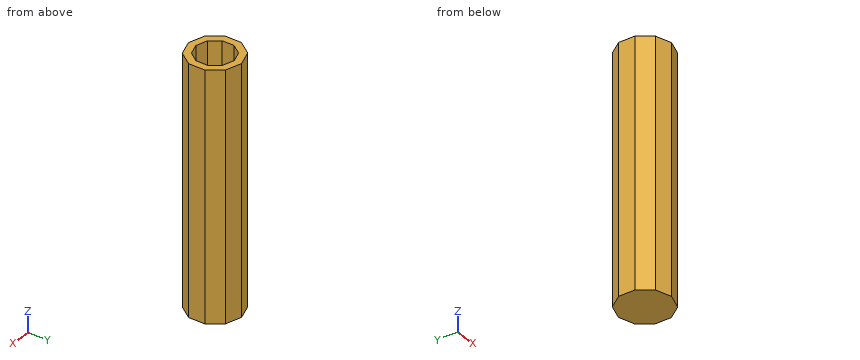
from build123d import *

# Parameters (mm, degrees)
F1_DEPTH = 381
F2_T     = -10.885714


with BuildPart() as f1:
    # F0 (on Top) → F1 (new body)
    with BuildSketch(Plane.XY):
        Polygon((39.086581, -12.7), (39.086581, 12.7), (24.156836, 33.249032), (0, 41.098063), (-24.156836, 33.249032), (-39.086581, 12.7), (-39.086581, -12.7), (-24.156836, -33.249032), (0, -41.098063), (24.156836, -33.249032), align=None)
    extrude(amount=F1_DEPTH)

    # F2
    f2_openings = [f1.faces().sort_by_distance(p)[0] for p in [
        (0, 0, 381),
    ]]
    offset(amount=F2_T, openings=f2_openings)


solid = f1.part
Input: part model. Units: mm. Frame: model coordinates. Give positions to 0.01 mm unless a question says otherwise; leave off trailing zeros. Order: outer loops, then holes, each group sorted by start corner. A loop starts at its lowest first (then second) coordinate and runs counter-clockwise, first axis right, second up. Notation, with made-up numbers: (-4, 23) -> (27, 23) arc R21 cw to (27, 55) -> close; hole circle Ø7 at (15.25, 4). An arc over 180 degrees is marked (long way). Use one line per item in the form item = value.
1) Section A-A, the plane z = 241. Return loops of the section in (x, y), and give its area (3 significant figures).
Response values:
outline = (-39.09, -12.7) -> (-24.16, -33.25) -> (0, -41.1) -> (24.16, -33.25) -> (39.09, -12.7) -> (39.09, 12.7) -> (24.16, 33.25) -> (0, 41.1) -> (-24.16, 33.25) -> (-39.09, 12.7) -> close; hole (-28.2, -9.16) -> (-17.43, -23.99) -> (0, -29.65) -> (17.43, -23.99) -> (28.2, -9.16) -> (28.2, 9.16) -> (17.43, 23.99) -> (0, 29.65) -> (-17.43, 23.99) -> (-28.2, 9.16) -> close
area = 2,380 mm^2
2) Line query: probe 1 along Z at (x, y) = (-26, 0.5); probe 2 along X at (y, z) = (-7, 155.5); probe 3 along Y at (x, z) = (-28, 72). Output: solid intervals per line, ascending.
Response values:
probe_1 = 0 to 10.89
probe_2 = -39.09 to -28.2, 28.2 to 39.09
probe_3 = -27.96 to -9.44, 9.44 to 27.96
3) First-contact query: pin 1 Ø5 at (y, z) = (-24.5, 318) entering from +X; pin 2 Ø1 at (x, z) = (18.5, 81.5) entering from +Y; pin 3 Ø10 at (y, z) = (-33, 92) entering from -X. Flat tips, straight axial feed; report the tip coordinate or a pass-through.
Response values:
pin_1 = 32.33
pin_2 = 35.25
pin_3 = -27.97
4) Section C-C, the plane x = 4.5. Return loops of the section in (y, z), and give its area (3 significant figures).
Response values:
outline = (-39.64, 0) -> (39.64, 0) -> (39.64, 381) -> (28.19, 381) -> (28.19, 10.89) -> (-28.19, 10.89) -> (-28.19, 381) -> (-39.64, 381) -> close
area = 9,340 mm^2
5) Section B-B, the plane y = 4.5. Return loops of the section in (x, z).
Response values:
outline = (-39.09, 0) -> (39.09, 0) -> (39.09, 381) -> (28.2, 381) -> (28.2, 10.89) -> (-28.2, 10.89) -> (-28.2, 381) -> (-39.09, 381) -> close
